Work out the finished part from the listing and answer in its coordinate system (mm). A direction names the side the tool comes from. Round coordinates to 2 decimals unless told otherwise and drop trailing zeros. Write each loop counter-clockwise with the first axis right and the second up, starting at its lowest first coordinate (ties: lowest second). Pieces come first, ordered by that corner, then holes. Notation, with made-up numbers: (56, 53.25) -> (99, 53.25) arc R20 cw to (99, 80.25) -> close; hole circle Ø4 at (6, 11). An arc over 180 degrees is marked (long way). Answer as a JSON object with one key per item and string values. Group by question number.
from build123d import *

# Parameters (mm, degrees)
F0_W     = 20.16
F0_H     = 20.16
F0_W_2   = 10
F0_H_2   = 10
F1_DEPTH = 88.9
F2_DEPTH = 50.8
F3_W     = 76.2
F3_H     = 2.54
F4_DEPTH = 330.2
F5_W     = 2.54
F5_H     = 76.2
F6_DEPTH = 190.5


with BuildPart() as f1:
    # F0 (on Front) → F1 (new body)
    with BuildSketch(Plane.XZ):
        with Locations((-204.3635635233, 0)):
            Rectangle(F0_W, F0_H)
        with Locations((-204.3635635233, 0)):
            Rectangle(F0_W_2, F0_H_2, mode=Mode.SUBTRACT)
        with Locations((-204.3635635233, 0)):
            Rectangle(F0_W_2, F0_H_2)
    extrude(amount=F1_DEPTH)


with BuildPart() as f1b:
    # F0 (on Front) → F1, piece 2 (new body)
    with BuildSketch(Plane.XZ):
        with Locations((145.9964364767, 0)):
            Rectangle(F0_W, F0_H)
        with Locations((145.9964364767, 0)):
            Rectangle(F0_W_2, F0_H_2, mode=Mode.SUBTRACT)
        with Locations((145.9964364767, 0)):
            Rectangle(F0_W_2, F0_H_2)
    extrude(amount=F1_DEPTH)


with BuildPart() as f2_tool:
    # F0 (on Front) → F2 (new body)
    with BuildSketch(Plane.XZ):
        with Locations((-204.3635635233, 0)):
            Rectangle(F0_W_2, F0_H_2)
        with Locations((145.9964364767, 0)):
            Rectangle(F0_W_2, F0_H_2)
    extrude(amount=F2_DEPTH)


with BuildPart() as f1_1:
    add(f1.part)

    # F2: cut by f2_tool
    add(f2_tool.part, mode=Mode.SUBTRACT)



with BuildPart() as f1b_1:
    add(f1b.part)

    # F2: cut by f2_tool
    add(f2_tool.part, mode=Mode.SUBTRACT)


with BuildPart() as f1_2:
    add(f1_1.part)

    add(f1b_1.part)  # F4 merges F1b
    # F3 (on face) → F4 (join, through all)
    with BuildSketch(Plane(origin=(135.9164364767, 0, 0), x_dir=(0, -1, 0), z_dir=(-1, 0, 0))):
        with Locations((44.45, 0)):
            Rectangle(F3_W, F3_H)
    extrude(amount=F4_DEPTH)

    # F5 (on face) → F6 (join)
    with BuildSketch(Plane.XY.offset(10.08)):
        with Locations((-204.3635635233, -44.45)):
            Rectangle(F5_W, F5_H)
        with Locations((145.9964364767, -44.45)):
            Rectangle(F5_W, F5_H)
    extrude(amount=F6_DEPTH)


solid = f1_2.part
1) Each of these flat-tipped pins is pushed along its axis until it touches: P1, Ø5, axis at y = -11.5, z = 142, coming from the +X side; P2, Ø1.3, axis at x = -85, z = 0, coming from the -Y side; P3, Ø10, axis at y = -57.5, z = 35, coming from the -X side. Where does it stop, or does it pass through?
2) For a pull along Z with two mould halves and no side action, classify faces 5 (the face through (-214.444, -44, 0)), 6 (the face through (146, -25, 5)), 7 (the face through (-27, -44, -1.27)) as released by +Z, released by -Z, zero draft, split by the parting line, or undercut.
3) A cutting plane is placed at D-D on x = -83. Determine the outline of the cut face in (y, z), plus the area to 3 significant figures.
4) A cutting plane is placed at B-B on y = -16. Determine the outline of the cut face in (x, z).
5) Straight lines are drawn through the part: L1, parallel to X at y = -60, z = 165; L2, parallel to Z at x = 3.5, y = -7. For each, find the intervals that lie inside material, in ascending order.
6) A cutting plane is placed at C-C on y = -66.5. Determine the outline of the cut face in (x, z), plus the area to 3 significant figures.
7) A tool of negligible diameter and unlimited length cuts with its end or side. For faces 1 (the face through (-27, -44, 1.27)), 2 (the face through (-205.634, -45, 104)), 3 (the face through (146, -25, -5)), 4 (the face through (153, 0, 0)), from which of +Z, -Z, +X, -X, +Y, -Y can it reach the whole face along a straight path? Write none if from no direction.
8) A cutting plane is placed at A-A on z = 84. Determine the outline of the cut face in (x, y), plus the area to 3 significant figures.
Established:
{
 "1": {"P1": "stops at x = 147.27", "P2": "stops at y = -82.55", "P3": "stops at x = -205.63"},
 "2": {"face 5": "zero draft", "face 6": "undercut", "face 7": "released by -Z"},
 "3": {"outline": "(-82.55, -1.27) -> (-6.35, -1.27) -> (-6.35, 1.27) -> (-82.55, 1.27) -> close", "area": "194 mm²"},
 "4": {"outline": "(-214.44, -10.08) -> (-194.28, -10.08) -> (-194.28, -1.27) -> (135.92, -1.27) -> (135.92, -10.08) -> (156.08, -10.08) -> (156.08, 10.08) -> (147.27, 10.08) -> (147.27, 200.58) -> (144.73, 200.58) -> (144.73, 10.08) -> (135.92, 10.08) -> (135.92, 1.27) -> (-194.28, 1.27) -> (-194.28, 10.08) -> (-203.09, 10.08) -> (-203.09, 200.58) -> (-205.63, 200.58) -> (-205.63, 10.08) -> (-214.44, 10.08) -> close; hole (-209.36, -5) -> (-199.36, -5) -> (-199.36, 5) -> (-209.36, 5) -> close; hole (141, -5) -> (151, -5) -> (151, 5) -> (141, 5) -> close"},
 "5": {"L1": "x = -205.63 to -203.09, 144.73 to 147.27", "L2": "z = -1.27 to 1.27"},
 "6": {"outline": "(-214.44, -10.08) -> (-194.28, -10.08) -> (-194.28, -1.27) -> (135.92, -1.27) -> (135.92, -10.08) -> (156.08, -10.08) -> (156.08, 10.08) -> (147.27, 10.08) -> (147.27, 200.58) -> (144.73, 200.58) -> (144.73, 10.08) -> (135.92, 10.08) -> (135.92, 1.27) -> (-194.28, 1.27) -> (-194.28, 10.08) -> (-203.09, 10.08) -> (-203.09, 200.58) -> (-205.63, 200.58) -> (-205.63, 10.08) -> (-214.44, 10.08) -> close", "area": "2,620 mm²"},
 "7": {"face 1": "+Z, +Y, -Y", "face 2": "+Z, -X, +Y, -Y", "face 3": "+Y", "face 4": "+Z, -Z, +X, -X, +Y"},
 "8": {"outline": "(-205.63, -82.55) -> (-203.09, -82.55) -> (-203.09, -6.35) -> (-205.63, -6.35) -> close; (144.73, -82.55) -> (147.27, -82.55) -> (147.27, -6.35) -> (144.73, -6.35) -> close", "area": "387 mm²"}
}
